Could you check a few things on this model? Use its own coordinates, in mm. A direction names the side the tool comes from. Give positions to 0.01 mm unless a question says otherwise; leave off trailing zeros. Order: outer loops, then holes, each group sorted by start corner. A loop starts at its lowest first (then second) coordinate and runs counter-clockwise, first axis right, second up. Notation, with made-up numbers: M 43,59 L 92,59 A33 cw 92,93 Z; hole C 79,35.5 d4. An arc over 180 degrees is marked long. Use a Markdown table: item, result. Add a question column.
Item 1: Suppose I cut it at D-D on x = 4. Write out the boundary of the cut face in (y, z), plus the area to 3 significant figures.
Item 2: Suppose I cut it at B-B on y = 5.35. Write out the boundary of the cut face in (x, z), plus the area to 3 significant figures.
Item 3: For faces 1 (the face through (-2, 2.25, 6)), 2 (the face through (22, 3, 3)), 3 (the face through (6.62, 1.11, -6.75)), which set-ups out of +Z, -Z, +X, -X, +Y, -Y let a thin tool reach every point of the face, with its end or its side?
Item 4: If I drill on L1, parallel to X at y = 3.25, z = 0; L2, parallel to X at y = 4.2, z = -3.5; L3, parallel to Z at x = -18.5, y = 2.55, over which ranges is the centre line in solid material (lowest first)? Write a range as from..to.
Item 5: Suppose I cut it at A-A on x = 17.5. Write out the boundary of the cut face in (y, z).
Item 6: Suppose I cut it at C-C on z = 4.5. Write out the boundary of the cut face in (x, y).
Item 7: I'm going to push flat-ended pins straight in: pin 1 Ø1.8 at (y, z) = (3, 10.55) entering from -X; pin 2 Ø5 at (x, z) = (1.5, -4.5) entering from +Y. Where does each tip first touch, or does it pass through?
Item 8: If we mould it in two halves opening along X, with no side actions, what happens to faces 4 (the face through (-24, 3, 3)), 5 (the face through (15, 3, -7.353)), 6 (the face through (6.05, 1, -3))? For each: released by +X, released by -X, zero draft, split by the parting line, or undercut.
from build123d import *

# Parameters (mm, degrees)
SKETCH3_R                   = 1.25
BOSS_EXTRUDE1_DEPTH         = 6
CUT_EXTRUDE1_DEPTH          = 3.75
M2_TAPPED_HOLE1_D           = 1.6
M2_TAPPED_HOLE1_DEPTH       = 8
M2_TAPPED_HOLE1_CSINK_D     = 2.05
M2_TAPPED_HOLE1_CSINK_ANGLE = 90
M2_TAPPED_HOLE1_TIP         = 0.480688495
M2_TAPPED_HOLE2_D           = 1.6
M2_TAPPED_HOLE2_DEPTH       = 8
M2_TAPPED_HOLE2_CSINK_D     = 2.05
M2_TAPPED_HOLE2_CSINK_ANGLE = 90
M2_TAPPED_HOLE2_TIP         = 0.480688495
M2_TAPPED_HOLE3_D           = 1.6
M2_TAPPED_HOLE3_DEPTH       = 6
M2_TAPPED_HOLE3_CSINK_D     = 2.05
M2_TAPPED_HOLE3_CSINK_ANGLE = 90
M2_TAPPED_HOLE3_TIP         = 0.480688495


with BuildPart() as part:
    # Sketch3 → Boss-Extrude1 (new body)
    with BuildSketch(Plane(origin=(0, 0, 0), x_dir=(1, 0, 0), z_dir=(0, 1, 0))):
        with BuildLine():
            Line((-24, 7.352825763), (-8.05, 7.352825763))
            ThreePointArc((-8.05, 7.352825763), (-6.635786438, 6.767039326), (-6.05, 5.352825763))
            Line((-6.05, 5.352825763), (-6.05, 0))
            ThreePointArc((-6.05, 0), (0, -6.05), (6.05, 0))
            Line((6.05, 0), (6.05, 5.352825763))
            ThreePointArc((6.05, 5.352825763), (6.635786438, 6.767039326), (8.05, 7.352825763))
            Line((8.05, 7.352825763), (22, 7.352825763))
            Line((22, 7.352825763), (22, -12.647174237))
            Line((22, -12.647174237), (-24, -12.647174237))
            Line((-24, -12.647174237), (-24, 7.352825763))
        make_face()
        with Locations(Location((-19.5, -8.147174237, 0), (0, 0, 270))):
            Circle(SKETCH3_R, mode=Mode.SUBTRACT)
        with Locations(Location((17.5, 4.352825763, 0), (0, 0, 270))):
            Circle(SKETCH3_R, mode=Mode.SUBTRACT)
        with Locations(Location((17.5, 0, 0), (0, 0, 270))):
            Circle(SKETCH3_R, mode=Mode.SUBTRACT)
        with Locations(Location((-19.5, 0, 0), (0, 0, 270))):
            Circle(SKETCH3_R, mode=Mode.SUBTRACT)
    extrude(amount=BOSS_EXTRUDE1_DEPTH)

    # Sketch6 → Cut-Extrude1 (cut)
    with BuildSketch(Plane(origin=(0, 6, 0), x_dir=(1, 0, 0), z_dir=(0, 1, 0))):
        with BuildLine():
            Line((-8.05, 0), (-8.05, 5.352825763))
            ThreePointArc((-8.05, 5.352825763), (-8.635786438, 6.767039326), (-10.05, 7.352825763))
            Line((-10.05, 7.352825763), (10.05, 7.352825763))
            ThreePointArc((10.05, 7.352825763), (8.635786438, 6.767039326), (8.05, 5.352825763))
            Line((8.05, 5.352825763), (8.05, 0))
            ThreePointArc((8.05, 0), (0, -8.05), (-8.05, 0))
        make_face()
    extrude(amount=-CUT_EXTRUDE1_DEPTH, mode=Mode.SUBTRACT)

    # M2 Tapped Hole1
    with Locations(Plane(origin=(22, 0, 0), x_dir=(0, 0, -1), z_dir=(1, 0, 0))):
        with Locations((-7.697174237, 3)):
            CounterSinkHole(M2_TAPPED_HOLE1_D / 2, M2_TAPPED_HOLE1_CSINK_D / 2, depth=M2_TAPPED_HOLE1_DEPTH, counter_sink_angle=M2_TAPPED_HOLE1_CSINK_ANGLE)
            with Locations((0, 0, -(M2_TAPPED_HOLE1_DEPTH + M2_TAPPED_HOLE1_TIP / 2))):  # 118° drill point
                Cone(0, M2_TAPPED_HOLE1_D / 2, M2_TAPPED_HOLE1_TIP, mode=Mode.SUBTRACT)

    # M2 Tapped Hole2
    with Locations(Plane.ZY.offset(24)):
        with Locations((10.547174237, 3)):
            CounterSinkHole(M2_TAPPED_HOLE2_D / 2, M2_TAPPED_HOLE2_CSINK_D / 2, depth=M2_TAPPED_HOLE2_DEPTH, counter_sink_angle=M2_TAPPED_HOLE2_CSINK_ANGLE)
            with Locations((0, 0, -(M2_TAPPED_HOLE2_DEPTH + M2_TAPPED_HOLE2_TIP / 2))):  # 118° drill point
                Cone(0, M2_TAPPED_HOLE2_D / 2, M2_TAPPED_HOLE2_TIP, mode=Mode.SUBTRACT)

    # M2 Tapped Hole3
    with Locations(Plane(origin=(0, 6, 0), x_dir=(1, 0, 0), z_dir=(0, 1, 0))):
        with Locations((-22.216954316, -6.30420158)):
            CounterSinkHole(M2_TAPPED_HOLE3_D / 2, M2_TAPPED_HOLE3_CSINK_D / 2, depth=M2_TAPPED_HOLE3_DEPTH, counter_sink_angle=M2_TAPPED_HOLE3_CSINK_ANGLE)
            with Locations((0, 0, -(M2_TAPPED_HOLE3_DEPTH + M2_TAPPED_HOLE3_TIP / 2))):  # 118° drill point
                Cone(0, M2_TAPPED_HOLE3_D / 2, M2_TAPPED_HOLE3_TIP, mode=Mode.SUBTRACT)


solid = part.part
Findings below:
| question | item | result |
|---|---|---|
| 1 | outline | M 0,4.54 L 2.25,4.54 L 2.25,6.99 L 6,6.99 L 6,12.65 L 0,12.65 Z |
| 1 | area | 39.5 mm^2 |
| 2 | outline | M -24,-7.35 L -10.05,-7.35 A2 ccw -8.05,-5.35 L -8.05,0 A8.05 cw 8.05,0 L 8.05,-5.35 A2 ccw 10.05,-7.35 L 22,-7.35 L 22,12.65 L -24,12.65 Z; hole C -22.22,6.3 d1.6; hole C -19.5,0 d2.5; hole C -19.5,8.15 d2.5; hole C 17.5,-4.35 d2.5; hole C 17.5,0 d2.5 |
| 2 | area | 676 mm^2 |
| 3 | face 1 | -Z, +Y |
| 3 | face 2 | +Z, -Z, +X, +Y, -Y |
| 3 | face 3 | -Z, +Y, -Y |
| 4 | L1 | x = -24..-20.75, -18.25..-8.05, 8.05..16.25, 18.75..22 |
| 4 | L2 | x = -24..-8.05, 8.05..16.59, 18.41..22 |
| 4 | L3 | z = -7.35..-0.75, 0.75..7.4, 8.9..9.89, 11.21..12.65 |
| 5 | outline | M 0,-7.35 L 6,-7.35 L 6,-5.6 L 0,-5.6 Z; M 0,-3.1 L 6,-3.1 L 6,-1.25 L 0,-1.25 Z; M 0,1.25 L 6,1.25 L 6,12.65 L 0,12.65 Z; hole C 3,7.7 d1.6 |
| 6 | outline | M -24,0 L -4.04,0 L -4.04,2.25 L -6.67,2.25 L -6.67,6 L -24,6 Z; M 4.04,0 L 22,0 L 22,6 L 6.67,6 L 6.67,2.25 L 4.04,2.25 Z |
| 7 | pin 1 | stops at x = -23.88 |
| 7 | pin 2 | passes through |
| 8 | face 4 | released by -X |
| 8 | face 5 | zero draft |
| 8 | face 6 | undercut |
